Geometry check sheet. Reference: the model listing, model coordinates, mm. A direction names the side the tool comes from. Give positions to 0.01 mm unless a question says otherwise; leave off trailing zeros. Write each loop counter-clockwise with the first axis right and the second up, starting at its lowest first coordinate (ties: lowest second). Pieces come first, ordered by that corner, then holes. Notation, with made-up numbers: (88, 81.25) - (102, 81.25) arc R17 cw to (102, 113.25) - close; hole circle Ø10 at (75.5, 26). An arc over 180 degrees is marked (long way). Write item = value, one per line. Start each with the question number.
(1) Depth check by flat-ended pin: pin 1 Ø4 at (x, y) = (11, 4) entering from +Z; pin 2 Ø5 at (x, y) = (-2, 1.5) entering from +Z; pin 3 Ø4.5 at (x, y) = (1, 0.5) entering from +Z. Enter the tip coordinate at first touch or a pass-through.
(2) Thickness scan on L1, parallel to Y at x = 0, z = 41.35; L2, parallel to Z at x = 5, y = -5.75; L3, parallel to X at y = 11.25, z = 31. Record the ranges inside material, lowest first.
(3) Draft check along X on faces 3 (the flat face through (0, 0, 40)), 4 (the cylindrical face through (18.797, -13.859, 20.224)), 5 (the cylindrical face through (-18.797, 13.859, 20.224)). Enter one of: pulls with the +X half, pulls with the -X half, needs draft (parallel to the pull), parting line crosses it, or undercut.
(4) Section check A-A, the plane x = -14. Enter the section's corners in (y, z).
(5) Access from +Z, -Z, +X, -X, +Y, -Y to the whole of each face (thin tool, end or side, straight path). Record for faces 1 (the cylindrical face through (-18.797, -0.154, 38.859)), 2 (the cylindrical face through (0, 2, 42)).
(6) Section check B-B, the plane y = 8.5. Enter the section's corners in (x, z).
Autodesk Inventor part; units mm, degrees
ref_plane "YZ Plane" through (0, 0, 0) normal (1, 0, 0) x (0, 1, 0)
ref_plane "XZ Plane" through (0, 0, 0) normal (0, 1, 0) x (-1, 0, 0)
ref_plane "XY Plane" through (0, 0, 0) normal (0, 0, 1) x (1, 0, 0)
sketch "Esboço1" plane through (0, 0, 0) normal (0, 0, 1) x (1, 0, 0)
  line L0 (-20, -15) -> (20, -15)
  line L1 (20, -15) -> (20, 15)
  line L2 (20, 15) -> (-20, 15)
  line L3 (-20, 15) -> (-20, -15)
  line L4 (-20, -15) -> (20, 15) construction
  line L5 (20, -15) -> (-20, 15) construction
  point P0 (0, 0)
  dimension "d0" = 30
  dimension "d1" = 40
extrude "Extrusão1" add sketch "Esboço1" along normal blind 40
fillet "Arredondamento1" radius 4 12 edges at (20, 0, 40) (0, 15, 40) (0, -15, 40) (-20, 0, 40) (-20, -15, 20) (-20, 0, 0) (0, 15, 0) (-20, 15, 20) (0, -15, 0) (20, 0, 0) (20, 15, 20) (20, -15, 20)
sketch "Esboço2" plane through (0, 0, 40) normal (0, 0, 1) x (1, 0, 0)
  circle A0 centre (0, 0) radius 5
  circle A1 centre (0, 0) radius 2
  dimension "d5" = 10
  dimension "d8" = 3
extrude "Extrusão2" add sketch "Esboço2" along normal blind 5 contours A0 | A1
extrude "Extrusão3" cut sketch "Esboço2" along normal blind 5 contours A1
chamfer "Chanfro1" distance 1.25 angle 45 1 edges at (-5, 0, 45)
chamfer "Chanfro2" distance 1.73 angle 45 1 edges at (-2, 0, 45)
properties part number "fonte IC"
Model answer:
q1.pin_1 = 40
q1.pin_2 = 45
q1.pin_3 = 44.64
q2.L1 = -5 to -2, 2 to 5
q2.L2 = 0 to 40
q2.L3 = -19.99 to 19.99
q3.face_3 = undercut
q3.face_4 = pulls with the +X half
q3.face_5 = pulls with the -X half
q4.outline = (-15, 4) arc R4 ccw to (-11, 0) - (11, 0) arc R4 ccw to (15, 4) - (15, 36) arc R4 ccw to (11, 40) - (-11, 40) arc R4 ccw to (-15, 36) - close
q5.face_1 = +Z, -X, +Y, -Y
q5.face_2 = +Z
q6.outline = (-20, 4) arc R4 ccw to (-16, 0) - (16, 0) arc R4 ccw to (20, 4) - (20, 36) arc R4 ccw to (16, 40) - (-16, 40) arc R4 ccw to (-20, 36) - close
